Autodesk Inventor part; units mm, degrees
ref_plane "YZ Plane" through (0, 0, 0) normal (1, 0, 0) x (0, 1, 0)
ref_plane "XZ Plane" through (0, 0, 0) normal (0, 1, 0) x (-1, 0, 0)
ref_plane "XY Plane" through (0, 0, 0) normal (0, 0, 1) x (1, 0, 0)
sketch "Sketch1" plane through (0, 0, 0) normal (0, 1, 0) x (-1, 0, 0)
  line L0 (0, 0) -> (127, 0)
  line L1 (127, 0) -> (127, -50.8)
  line L2 (127, -50.8) -> (0, -50.8)
  line L3 (0, -50.8) -> (0, 0)
  dimension "d0" = 127
  dimension "d1" = 50.8
extrude "Extrusion1" add sketch "Sketch1" along normal blind 38.1
sketch "Sketch2" plane through (-127, 0, 0) normal (0, 0, 1) x (1, 0, 0)
  line L0 (123.825, 0) -> (3.175, 0) construction
  circle A0 centre (63.4683, 18.9303) radius 6.985
  circle A1 centre (12.6683, 18.9303) radius 6.985
  circle A2 centre (114.2683, 18.9303) radius 6.985
  line L1 (63.5, 0) -> (63.5, 25.2805) construction
  line L2 (127, 0) -> (127, 38.1) construction
  line L3 (127, 19.05) -> (0, 19.05) construction
  point P0 (0, -12.7)
  dimension "d4" = 13.97
  dimension "d5" = 13.97
  dimension "d8" = 13.97
  dimension "d9" = 50.8
  dimension "d10" = 50.8
extrude "Extrusion2" cut sketch "Sketch2" against normal through all
sketch "Sketch3" plane through (-127, 0, 0) normal (0, 0, 1) x (1, 0, 0)
  circle A0 centre (63.4683, 18.9303) radius 6.985
  line L0 (63.4683, 31.7619) -> (74.5808, 25.3461)
  line L1 (74.5808, 25.3461) -> (74.5808, 12.5145)
  line L2 (74.5808, 12.5145) -> (63.4683, 6.0987)
  line L3 (63.4683, 6.0987) -> (52.3558, 12.5145)
  line L4 (52.3558, 12.5145) -> (52.3558, 25.3461)
  line L5 (52.3558, 25.3461) -> (63.4683, 31.7619)
  point P0 (127, 0)
  dimension "d11" = 22.225
extrude "Extrusion3" cut sketch "Sketch3" against normal blind 12.7
sketch "Sketch4" plane through (0, 0, -50.8) normal (0, 0, -1) x (-1, 0, 0)
  line L0 (63.4683, 31.7619) -> (74.5808, 25.3461)
  line L1 (74.5808, 25.3461) -> (74.5808, 12.5145)
  line L2 (74.5808, 12.5145) -> (63.4683, 6.0987)
  line L3 (63.4683, 6.0987) -> (52.3558, 12.5145)
  line L4 (52.3558, 12.5145) -> (52.3558, 25.3461)
  line L5 (52.3558, 25.3461) -> (63.4683, 31.7619)
  point P0 (0, 0)
  point P1 (127, 0)
  point P2 (63.4683, 18.9303)
  dimension "d14" = 22.225
extrude "Extrusion5" cut sketch "Sketch4" against normal blind 12.7
sketch "Sketch5" plane through (0, 0, 0) normal (0, -1, 0) x (1, 0, 0)
  line L0 (-63.4683, -50.8) -> (-66.6433, -50.8)
  line L1 (-66.6433, -50.8) -> (-66.6433, 0)
  line L2 (-66.6433, 0) -> (-63.4683, 0)
  line L3 (-63.4683, 0) -> (-63.4683, -50.8) construction
  line L4 (-63.4683, -50.8) -> (-60.2933, -50.8)
  line L5 (-60.2933, -50.8) -> (-60.2933, 0)
  line L6 (-60.2933, 0) -> (-63.4683, 0)
  point P0 (0, 0)
  dimension "d19" = 3.175
  dimension "d20" = 50.8
extrude "Extrusion6" add sketch "Sketch5" along normal blind 101.6
sketch "Sketch6" plane through (-66.6433, 0, -50.8) normal (-1, 0, 0) x (0, 0, 1)
  line L0 (0, 0) -> (0, -101.6) construction
  line L1 (0, -101.6) -> (50.8, -101.6) construction
  line L2 (50.8, -101.6) -> (50.8, -50.8) construction
  line L3 (50.8, -50.8) -> (0, -50.8) construction
  line L4 (0, -50.8) -> (0, -101.6) construction
  line L5 (0, -50.8) -> (49.9098, -101.6) construction
  line L6 (9.0799, -92.075) -> (40.8299, -92.075) construction
  line L7 (40.8299, -92.075) -> (40.8299, -60.325) construction
  line L8 (40.8299, -60.325) -> (9.0799, -60.325) construction
  line L9 (9.0799, -60.325) -> (9.0799, -92.075) construction
  line L10 (9.0799, -92.075) -> (40.8299, -60.325) construction
  line L11 (40.8299, -92.075) -> (9.0799, -60.325) construction
  circle A0 centre (40.8299, -60.325) radius 3.175
  circle A1 centre (40.8299, -92.075) radius 3.175
  circle A2 centre (9.0799, -92.075) radius 3.175
  circle A3 centre (9.0799, -60.325) radius 3.175
  point P0 (50.8, 0)
  point P1 (24.9549, -76.2)
  dimension "d23" = 50.8
  dimension "d24" = 50.8
  dimension "d25" = 31.75
  dimension "d26" = 31.75
  dimension "d27" = 6.35
  dimension "d28" = 6.35
  dimension "d29" = 6.35
  dimension "d30" = 6.35
extrude "Extrusion7" cut sketch "Sketch6" against normal through all
properties part number "Traveller"
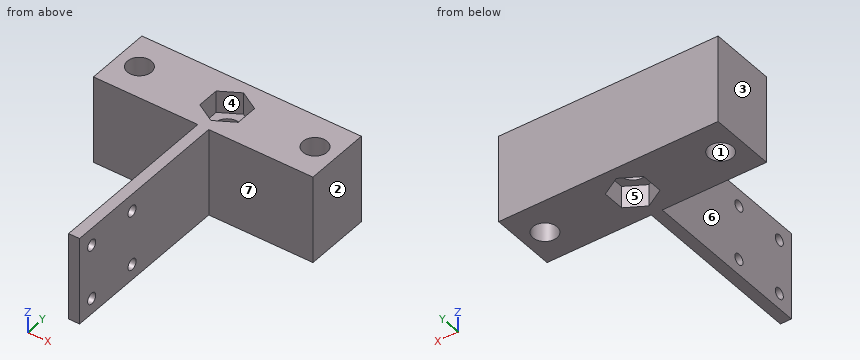
The model under review builds one solid part; all positions refer to its coordinate system, in mm. Face numbers are marked on the shaded views. A direction names the side the tool comes from. Coordinates: 2 decimals unless noted, no trailing zeros. Order: outer loops, then holes, each group sorted by start corner. A loop starts at its lowest first (then second) coordinate and runs counter-clockwise, first axis right, second up. Notation, with made-up numbers: (45.25, -2.5) -> (74.25, -2.5) arc R14 cw to (74.25, 14.5) -> close; hole circle Ø4 at (-25.5, -9.5). An arc over 180 degrees is marked (long way). Answer in a Markdown table with one row per item.
(1) Consider section A-A (y = 8.5). Write out the cut boundary in (x, z).
Answers:
| item | result |
|---|---|
| outline | (-127, -50.8) -> (-67.63, -50.8) -> (-67.63, -38.1) -> (-59.31, -38.1) -> (-59.31, -50.8) -> (0, -50.8) -> (0, 0) -> (-59.37, 0) -> (-59.37, -12.7) -> (-67.69, -12.7) -> (-67.69, 0) -> (-127, 0) -> close |
(2) Consider section B-B (z = -22). Write out the cut boundary in (x, y) (3 decimals), plus the area to 3 significant figures.
Answers:
| item | result |
|---|---|
| outline | (-127, 0) -> (-66.643, 0) -> (-66.643, -101.6) -> (-60.293, -101.6) -> (-60.293, 0) -> (0, 0) -> (0, 38.1) -> (-127, 38.1) -> close; hole circle Ø13.97 at (-114.332, 18.93); hole circle Ø13.97 at (-63.532, 18.93); hole circle Ø13.97 at (-12.732, 18.93) |
| area | 5,020 mm² |
(3) The part is to be moulded in two halves that separate along X. For the marked faces 1, 2 and 3, say which applies: +X half, -X half, draft (parallel to the pull), parting line (faces both ways), or undercut.
Answers:
| item | result |
|---|---|
| face 1 | undercut |
| face 2 | +X half |
| face 3 | -X half |
(4) Consider section C-C (x = -88). Write out the cut boundary in (y, z).
Answers:
| item | result |
|---|---|
| outline | (0, -50.8) -> (38.1, -50.8) -> (38.1, 0) -> (0, 0) -> close |
(5) Wall thickness on line 1 along Z through (x, y) = (-63, -90.5); line 2 along Y through (x, z) = (-45, -39.5); line 3 along X through (y, z) = (-12, -42): over which ranges is each line inside the solid? List them lowest first.
Answers:
| item | result |
|---|---|
| line 1 | -50.8 to -44.48, -38.96 to -12.73, -7.21 to 0 |
| line 2 | 0 to 38.1 |
| line 3 | -66.64 to -60.29 |
(6) Machinability: for the marked faces 4, 5, 6 and 7, which of the approach directions +Z, -Z, +X, -X, +Y, -Y give a long, thin tool a straight path to every point of the face, cutting with its end or side? Answer none if there is none.
Answers:
| item | result |
|---|---|
| face 4 | +Z |
| face 5 | -Z |
| face 6 | +Z, -Z, -X, -Y |
| face 7 | +Z, -Z, +X, -Y |
(7) Insertion check: pin 1 (10 mm diameter, centred on y = -60.32, z = -41.72, fed in from +X); pin 2 (12 mm diameter, centred on x = -82, z = -43.5, fed in from -Y); pin 3 (15 mm diameter, centred on y = -51, z = -23.5, fed in from -X); pin 4 (18 mm diameter, centred on x = -65.5, y = 15.5, fed in from -Z). Each pin has a flat end and moves straight along its axis. Give the tip position at first contact, or say it passes through.
Answers:
| item | result |
|---|---|
| pin 1 | x = -60.29 |
| pin 2 | y = 0 |
| pin 3 | x = -66.64 |
| pin 4 | z = -50.8 |
